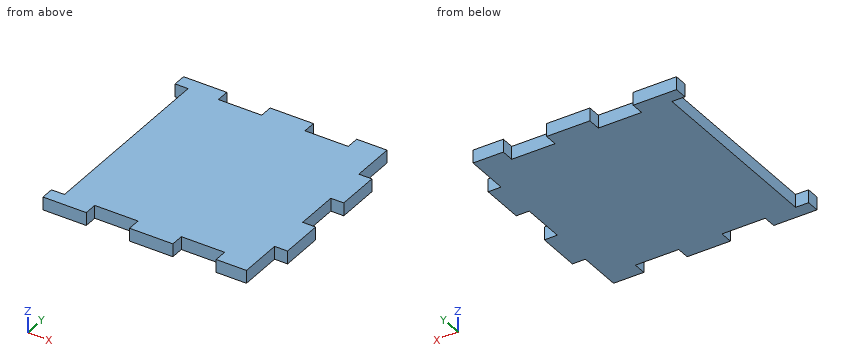
```python
from build123d import *

# Parameters (mm, degrees)
SKETCH1_W           = 50
SKETCH1_H           = 50
BOSS_EXTRUDE1_DEPTH = 3
SKETCH2_W           = 10
SKETCH2_H           = 3
SKETCH2_W_2         = 3
SKETCH2_H_2         = 10
CUT_EXTRUDE1_DEPTH  = 3
CAVITY1_START       = -22
CAVITY1_OUTLINE_W   = 3
CAVITY1_OUTLINE_H   = 3
CAVITY1_DEPTH       = 44


# Read off the part's stored shape, not the designer's step: Cavity1
with BuildPart() as part:
    # Sketch1 → Boss-Extrude1 (new body)
    with BuildSketch(Plane.XY):
        Rectangle(SKETCH1_W, SKETCH1_H)
    extrude(amount=BOSS_EXTRUDE1_DEPTH)

    # Sketch2 → Cut-Extrude1 (cut)
    with BuildSketch(Plane.XY.offset(3)):
        with Locations((-10, 23.5)):
            Rectangle(SKETCH2_W, SKETCH2_H)
        with Locations((10, 23.5)):
            Rectangle(SKETCH2_W, SKETCH2_H)
        with Locations((10, -23.5)):
            Rectangle(SKETCH2_W, SKETCH2_H)
        with Locations((-10, -23.5)):
            Rectangle(SKETCH2_W, SKETCH2_H)
        with Locations((23.5, 20)):
            Rectangle(SKETCH2_W_2, SKETCH2_H_2)
        with Locations((23.5, -20)):
            Rectangle(SKETCH2_W_2, SKETCH2_H_2)
        with Locations((23.5, 0)):
            Rectangle(SKETCH2_W_2, SKETCH2_H_2)
    extrude(amount=-CUT_EXTRUDE1_DEPTH, mode=Mode.SUBTRACT)

    # Cavity1 outline → Cavity1 (cut)
    with BuildSketch(Plane(origin=(0, 0, 0), x_dir=(1, 0, 0), z_dir=(0, 1, 0)).offset(CAVITY1_START)):
        with Locations((-23.5, -1.5)):
            Rectangle(CAVITY1_OUTLINE_W, CAVITY1_OUTLINE_H)
    extrude(amount=CAVITY1_DEPTH, mode=Mode.SUBTRACT)


solid = part.part
```
Check sheet for the modelled part. Datum: model origin and axes. Units: mm. Coordinates: 2 decimals unless noted, no trailing zeros. Write each loop counter-clockwise with the first axis right and the second up, starting at its lowest first coordinate (ties: lowest second). Pieces come first, ordered by that corner, then holes. Notation, with made-up numbers: (21.25, -9.75) -> (65.25, -9.75) arc R21 ccw to (65.25, 14.25) -> close; hole circle Ø3 at (-25, 7.5). An arc over 180 degrees is marked (long way). Use a Markdown table: item, result.
1. Go/stop test with flat-tipped pins: pin 1 Ø0.9 at (x, z) = (-11.5, 1) entering from -Y; pin 2 Ø0.9 at (x, z) = (23, 1.5) entering from +Y; pin 3 Ø0.9 at (y, z) = (-1, 1) entering from -X. Record where each tip stops, or that it passes through.
Reported:
| item | result |
|---|---|
| pin 1 | stops at y = -22 |
| pin 2 | stops at y = 15 |
| pin 3 | stops at x = -22 |
2. Scan lines: line 1 along X through (y, z) = (16, 0.65); line 2 along X through (y, z) = (11, 0.85). Record each from-to range of solid material in increasing order.
Reported:
| item | result |
|---|---|
| line 1 | x = -22 to 22 |
| line 2 | x = -22 to 25 |
3. Sectioned sample at C-C (x = -9). Enter the section's corners in (y, z).
Reported:
| item | result |
|---|---|
| outline | (-22, 0) -> (22, 0) -> (22, 3) -> (-22, 3) -> close |
4. Sectioned sample at B-B (y = -12.5). Enter the section's corners in (x, z), plus the area to 3 significant figures.
Reported:
| item | result |
|---|---|
| outline | (-22, 0) -> (25, 0) -> (25, 3) -> (-22, 3) -> close |
| area | 141 mm2 |
